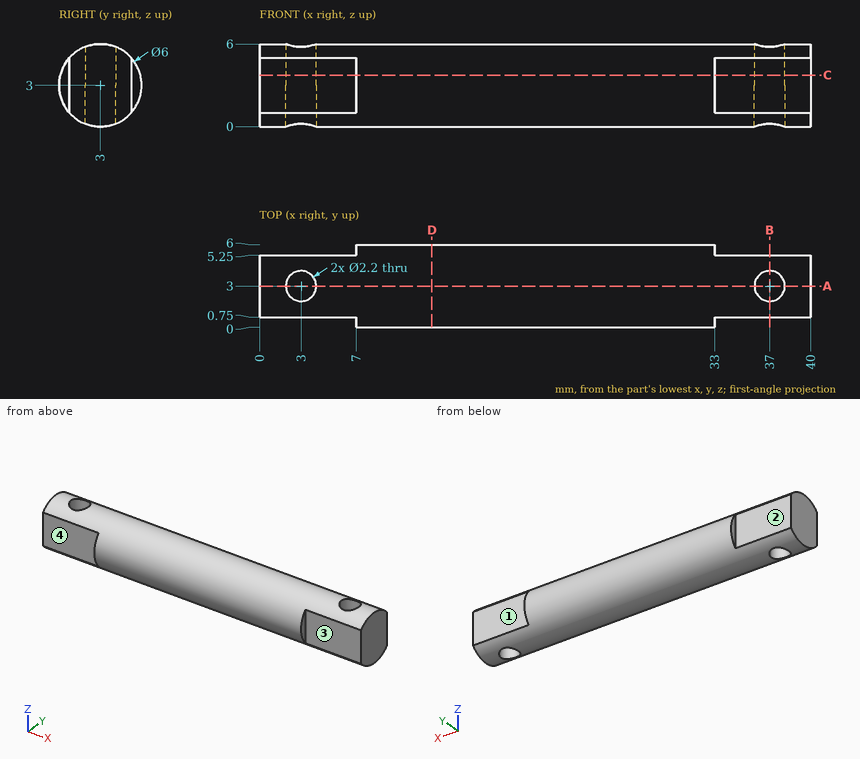
Print and shaded views of the part. All mm, measured from the part's lowest x, y and z. A direction names the side the tool comes from. Coordinates: 2 decimals unless noted, no trailing zeros. Order: outer loops, then holes, each group sorted by start corner. A loop starts at its lowest first (then second) coordinate and runs counter-clockwise, first axis right, second up. Notation, with made-up numbers: (44.25, 74) -> (74.25, 74) arc R20 cw to (74.25, 88) -> close; hole circle Ø5 at (68.5, 57). An arc over 180 degrees is marked (long way). Use one line per item in the form item = value. Start each with the question number.
1) Band-saw the part on A-A on y = 3. Give the cut face in (x, z).
2) Tool access for the marked faces 1, 2, 3 and 4: list every direction of +Z, -Z, +X, -X, +Y, -Y with a clear straight run to the whole face (end or side of a thin tool).
3) Band-saw the part on B-B on x = 37. Give the cut face in (y, z).
4) Band-saw the part on C-C on z = 3.75. Give the cut face in (x, y), then the cut area to 3 significant figures.
5) Drill centre lines: L1, parallel to Y at x = 3, z = 1.2; L2, parallel to X at y = 2.25, z = 2.25; L3, parallel to X at y = 3.5, z = 0.5. Where is each one in solid material? Low to high. Write a range as [from, to].
6) Band-saw the part on D-D on x = 12.5. Give the cut face in (y, z), then the cut area to 3 significant figures.
7) Drop flat-ended pins along their axis: pin 1 (2 mm diameter, centred on x = 21, z = 5, fed in from -Y); pin 2 (2.5 mm diameter, centred on x = 37, y = 3, fed in from -Z); pin 3 (2 mm diameter, centred on x = 2.5, z = 2, fed in from +Y); pin 4 (1.2 mm diameter, centred on x = 2, z = 2.5, fed in from -Y). Give the stop position or say it passes through.
Entries:
q1.outline = (0, 0) -> (1.9, 0) -> (1.9, 6) -> (0, 6) -> close; (4.1, 0) -> (35.9, 0) -> (35.9, 6) -> (4.1, 6) -> close; (38.1, 0) -> (40, 0) -> (40, 6) -> (38.1, 6) -> close
q2.face_1 = +Z, -Z, +X, +Y
q2.face_2 = +Z, -Z, -X, +Y
q2.face_3 = +Z, -Z, +X, -Y
q2.face_4 = +Z, -Z, -X, -Y
q3.outline = (0.75, 1.02) arc R3 ccw to (1.9, 0.21) -> (1.9, 5.79) arc R3 ccw to (0.75, 4.98) -> close; (4.1, 0.21) arc R3 ccw to (5.25, 1.02) -> (5.25, 4.98) arc R3 ccw to (4.1, 5.79) -> close
q4.outline = (0, 0.75) -> (7, 0.75) -> (7, 0.1) -> (33, 0.1) -> (33, 0.75) -> (40, 0.75) -> (40, 5.25) -> (33, 5.25) -> (33, 5.9) -> (7, 5.9) -> (7, 5.25) -> (0, 5.25) -> close; hole circle Ø2.2 at (3, 3); hole circle Ø2.2 at (37, 3)
q4.area = 206 mm2
q5.L1 = [0.75, 1.9], [4.1, 5.25]
q5.L2 = [0, 2.2], [3.8, 36.2], [37.8, 40]
q5.L3 = [0, 2.02], [3.98, 36.02], [37.98, 40]
q6.outline = circle Ø6 at (3, 3)
q6.area = 28.3 mm2
q7.pin_1 = 0.17
q7.pin_2 = 0
q7.pin_3 = 5.25
q7.pin_4 = 0.75
